```python
from build123d import *

# Parameters (mm, degrees)
PAD_DEPTH = 2


with BuildPart() as part:
    # Sketch → Pad (new body)
    with BuildSketch(Plane.XZ):
        Polygon((-0.507831, 0.029803), (-0.507831, 110.029803), (11.492169, 110.029803), (11.492169, 122.029803), (171.492169, 122.029803), (171.492169, 110.029803), (156.492169, 110.029803), (156.492169, 20.029803), (11.492169, 20.029803), (11.492169, 0.029803), align=None)
    extrude(amount=PAD_DEPTH)


solid = part.part
```
CAD build for the part. Positions are in the model's coordinates, mm. Round coordinates to 2 decimals unless told otherwise and drop trailing zeros. Order: outer loops, then holes, each group sorted by start corner. A loop starts at its lowest first (then second) coordinate and runs counter-clockwise, first axis right, second up. Notation, with made-up numbers: (78.25, 29) - (93.25, 29) arc R15 cw to (93.25, 34) - close; hole circle Ø3 at (-2, -6.5). An arc over 180 degrees is marked (long way). Answer as CSV lines item,"result". Start each with the question number.
1. Pin check, flat tips, straight feed: pin 1 (1 mm diameter, centred on y = -0.5, z = 6, fed in from +X); pin 2 (0.6 mm diameter, centred on x = 8, y = -1.5, fed in from +Z); pin 3 (12 mm diameter, centred on x = 43.5, z = 27, fed in from +Y). Stop position of each tip, or through.
2. Saw through at A-A, the plane y = -0.85. Write the cut outline in (x, z).
3. Saw through at B-B, the plane z = 112.5. Write the cut outline in (x, y).
4. Saw through at C-C, the plane x = 80.5. Write the cut outline in (y, z), and give its area (3 significant figures).
5. Drill centre lines: L1, parallel to Z at x = 57.5, y = -0.2; L2, parallel to X at y = -1.7, z = 9; L3, parallel to X at y = -1.5, z = 83. Where is each one in solid material? Low to high. Write a range as [from, to].
Model answer:
1,pin 1,"stops at x = 11.49"
1,pin 2,"stops at z = 110.03"
1,pin 3,"stops at y = 0"
2,outline,"(-0.51, 0.03) - (11.49, 0.03) - (11.49, 20.03) - (156.49, 20.03) - (156.49, 110.03) - (171.49, 110.03) - (171.49, 122.03) - (11.49, 122.03) - (11.49, 110.03) - (-0.51, 110.03) - close"
3,outline,"(11.49, -2) - (171.49, -2) - (171.49, 0) - (11.49, 0) - close"
4,outline,"(-2, 20.03) - (0, 20.03) - (0, 122.03) - (-2, 122.03) - close"
4,area,"204 mm²"
5,L1,"z = [20.03, 122.03]"
5,L2,"x = [-0.51, 11.49]"
5,L3,"x = [-0.51, 156.49]"
